Could you check a few things on this model? Use its own coordinates, in mm. A direction names the side the tool comes from. Give positions to 0.01 mm unless a question says otherwise; leave off trailing zeros. Order: outer loops, then holes, each group sorted by start corner. A loop starts at its lowest first (then second) coordinate and runs counter-clockwise, first axis right, second up. Notation, with made-up numbers: M 58.5,-39.75 L 89.5,-39.75 A29 ccw 89.5,-17.75 Z; hole C 39.5,-3 d10. An arc over 180 degrees is marked long. Use a Markdown table: item, result. Add a question column.
Item 1: Suppose I cut it at A-A on x = 0. Write out the boundary of the cut face in (y, z).
Item 2: If I drill on L1, parallel to Y at x = 0, z = 12; L2, parallel to X at y = -6, z = 81; L3, parallel to X at y = -1, z = 57, over which ranges is the centre line in solid material (lowest first)? Write a range as from..to.
Item 3: Suppose I cut it at C-C on y = 0. Count the separate pieces of the cut face and the enclosed holes in it, plus the area to 3 significant figures.
Item 4: For faces 1 (the face through (-42, 0, 130)), 2 (the face through (-20, 1, 84)), 3 (the face through (-22, 0, 150)), 4 (the face through (36, 0, 128)), which set-ups out of +Z, -Z, +X, -X, +Y, -Y let a thin tool reach every point of the face, with its end or its side?
Item 5: I'm going to push flat-ended pins straight in: pin 1 Ø12 at (x, y) = (5.5, -15.5) entering from +Z; pin 2 Ø12 at (y, z) = (-23.5, 16.5) entering from -X; pin 3 Ø4 at (y, z) = (-34.5, 132.5) entering from +X. Where does each tip first touch, or does it pass through?
Item 6: Suppose I cut it at B-B on z = 100. Write out the boundary of the cut face in (x, y), plus the area to 3 significant figures.
Item 7: Suppose I cut it at D-D on z = 63. Write out the boundary of the cut face in (x, y), plus the area to 3 significant figures.
Item 8: If we mould it in two halves opening along Y, with no side actions, what happens to faces 5 (the face through (42, 0, 70)), 6 (the face through (11.923, 3.755, 9.86)), 7 (the face through (27.605, -1.302, 109.915)), 8 (the face through (24.192, 37.944, 49.646))? For each: released by +Y, released by -Y, zero draft, split by the parting line, or undercut.
from build123d import *

# Parameters (mm, degrees)
F0_R          = 45
F0_R_2        = 12.5
F1_DEPTH      = 150
F2_W          = 40
F2_H          = 150
F2_W_2        = 22.3551505804
F2_H_2        = 60
F3_DEPTH      = 100
F3_DEPTH_BACK = 100
F4_R          = 19.99999
F5_R          = 5
F6_R          = 10
F7_DEPTH      = 150


# Not quite as in the source:
# - a fillet or chamfer is up to 0.001 mm smaller than in the source, because OpenCascade refuses the exact size


with BuildPart() as f1:
    # F0 (on Top) → F1 (new body)
    with BuildSketch(Plane.XY):
        Circle(F0_R)
        Circle(F0_R_2, mode=Mode.SUBTRACT)
    extrude(amount=F1_DEPTH)

    # F2 (on Front) → F3 (cut, two sides)
    with BuildSketch(Plane.XZ) as f3_sk:
        with Locations((0, 95)):
            Rectangle(F2_W, F2_H)
        with Locations((-46.1775752902, 100)):
            Rectangle(F2_W_2, F2_H_2)
        with Locations((46.1775752902, 100)):
            Rectangle(F2_W_2, F2_H_2)
    extrude(amount=-F3_DEPTH, mode=Mode.SUBTRACT)
    extrude(f3_sk.sketch, amount=F3_DEPTH_BACK, mode=Mode.SUBTRACT)

    # F4 (radius 20 in the source; OpenCascade refuses exactly that, so slightly less here)
    f4_edges = [f1.edges().sort_by_distance(p)[0] for p in [
        (-45, 0, 150),
        (38.242646, -23.717082, 150),
        (38.242646, 23.717082, 150),
    ]]
    fillet(f4_edges, radius=F4_R)

    # F5
    f5_edges = [f1.edges().sort_by_distance(p)[0] for p in [
        (-35, 0, 130),
        (-35, 0, 70),
        (35, 0, 70),
        (35, 0, 130),
    ]]
    fillet(f5_edges, radius=F5_R)

    # F6 (on face) → F7 (cut)
    with BuildSketch(Plane.YZ.offset(35)):
        with Locations((0, 100)):
            Circle(F6_R)
    extrude(amount=-F7_DEPTH, mode=Mode.SUBTRACT)


solid = f1.part
Findings below:
| question | item | result |
|---|---|---|
| 1 | outline | M -45,0 L -12.5,0 L -12.5,20 L -45,20 Z; M 12.5,0 L 45,0 L 45,20 L 12.5,20 Z |
| 2 | L1 | y = -45..-12.5, 12.5..45 |
| 2 | L2 | x = -35..-20, 20..35 |
| 2 | L3 | x = -44.99..-20, 20..44.99 |
| 3 | separate pieces | 4 |
| 3 | enclosed holes | 0 |
| 3 | area | 5,850 mm^2 |
| 4 | face 1 | -X, +Y, -Y |
| 4 | face 2 | +Z, +Y, -Y |
| 4 | face 3 | +Z, +X, -X, +Y, -Y |
| 4 | face 4 | +X, +Y, -Y |
| 5 | pin 1 | stops at z = 20 |
| 5 | pin 2 | stops at x = -41.46 |
| 5 | pin 3 | stops at x = 30.93 |
| 6 | outline | M -35,-28.28 A45 ccw -20,-40.31 L -20,-10 L -35,-10 Z; M -35,10 L -20,10 L -20,40.31 A45 ccw -35,28.28 Z; M 20,-40.31 A45 ccw 35,-28.28 L 35,-10 L 20,-10 Z; M 20,10 L 35,10 L 35,28.28 A45 ccw 20,40.31 Z |
| 6 | area | 1,510 mm^2 |
| 7 | outline | M -20,-40.31 L -20,40.31 A45 ccw Z; M 20,-40.31 A45 ccw 20,40.31 Z |
| 7 | area | 2,880 mm^2 |
| 8 | face 5 | zero draft |
| 8 | face 6 | undercut |
| 8 | face 7 | undercut |
| 8 | face 8 | split by the parting line |
